Source: CAD feature listing. Evaluate the final solid. Frame: model axes, mm. Face numbers are marked on the shaded views. A direction names the side the tool comes from. Coordinates: 2 decimals unless noted, no trailing zeros. Order: outer loops, then holes, each group sorted by start corner. A loop starts at its lowest first (then second) coordinate and runs counter-clockwise, first axis right, second up.
```python
from build123d import *

# Parameters (mm, degrees)
SKETCH4_R           = 2
SKETCH4_R_2         = 3.96875
BOSS_EXTRUDE2_DEPTH = 6.35
FILLET1_R           = 5.08
FILLET7_R           = 3.81
FILLET9_R           = 5.08
FILLET10_R          = 1.27
FILLET11_R          = 3.81
FILLET12_R          = 2.54
FILLET13_R          = 3.81


with BuildPart() as part:
    # Sketch4 → Boss-Extrude2 (new body)
    with BuildSketch(Plane(origin=(0, 0, 0), x_dir=(1, 0, 0), z_dir=(0, 1, 0))):
        with BuildLine():
            Line((22.483900583, -18.4375), (28.735494078, -18.4375))
            Line((28.735494078, -18.4375), (48.985566477, 12.027918285))
            Line((48.985566477, 12.027918285), (54.680415238, 16.319294633))
            ThreePointArc((54.680415238, 16.319294633), (55.797199918, 17.662082259), (56.1975, 19.362095927))
            Line((56.1975, 19.362095927), (56.1975, 26.9875))
            ThreePointArc((56.1975, 26.9875), (55.081576836, 29.681576836), (52.3875, 30.7975))
            Line((52.3875, 30.7975), (-4.7625, 30.7975))
            ThreePointArc((-4.7625, 30.7975), (-7.456576836, 29.681576836), (-8.5725, 26.9875))
            Line((-8.5725, 26.9875), (-8.5725, 12.607500122))
            Line((-8.5725, 12.607500122), (-8.5725, 0.508))
            Line((-8.5725, 0.508), (-23.52171402, 0.508))
            Line((-23.52171402, 0.508), (-23.52171402, -9.652))
            Line((-23.52171402, -9.652), (-14.139296969, -9.652))
            Line((-14.139296969, -9.652), (-23.148009155, -20.371437257))
            Line((-23.148009155, -20.371437257), (-17.314513469, -25.273959881))
            Line((-17.314513469, -25.273959881), (-11.569090649, -18.4375))
            Line((-11.569090649, -18.4375), (22.483900583, -18.4375))
        make_face()
        with Locations(Location((-17.78, -19.905950726, 0), (0, 0, 270))):
            Circle(SKETCH4_R, mode=Mode.SUBTRACT)
        with BuildLine():
            ThreePointArc((-16.29541402, -4.572), (-20.572189245, -4.832151892), (-16.358479767, -4.055532442))
            ThreePointArc((-16.358479767, -4.055532442), (-16.311238795, -4.311848108), (-16.29541402, -4.572))
        make_face(mode=Mode.SUBTRACT)
        with BuildLine():
            ThreePointArc((-7.62, -15.8975), (-10.16, -13.3575), (-7.62, -10.8175))
            Line((-7.62, -10.8175), (12.7, -10.8175))
            Line((12.7, -10.8175), (12.7, -5.7375))
            ThreePointArc((12.7, -5.7375), (15.24, -3.1975), (17.78, -5.7375))
            Line((17.78, -5.7375), (17.78, -13.3575))
            Line((17.78, -13.3575), (17.78, -15.8975))
            Line((17.78, -15.8975), (15.24, -15.8975))
            Line((15.24, -15.8975), (-7.62, -15.8975))
        make_face(mode=Mode.SUBTRACT)
        with BuildLine():
            ThreePointArc((-6.163414949, -1.528010526), (-1.528010526, 6.163414949), (6.163414949, 1.528010526))
            ThreePointArc((6.163414949, 1.528010526), (6.303181138, 0.769680153), (6.35, 0))
            ThreePointArc((6.35, 0), (0.769680153, -6.303181138), (-6.163414949, -1.528010526))
        make_face(mode=Mode.SUBTRACT)
        with Locations(Location((24.012521227, -14.703599027, 0), (0, 0, 270))):
            Circle(SKETCH4_R, mode=Mode.SUBTRACT)
        with Locations(Location((-1.5875, 21.9075, 0), (0, 0, 270))):
            Circle(SKETCH4_R_2, mode=Mode.SUBTRACT)
        with BuildLine():
            ThreePointArc((20.58801402, 4.572), (18.701865912, 2.441524775), (16.358479767, 4.055532442))
            ThreePointArc((16.358479767, 4.055532442), (18.181562129, 6.702475225), (20.58801402, 4.572))
        make_face(mode=Mode.SUBTRACT)
        Polygon((6.749565973, 9.2075), (6.749565973, 26.9875), (40.692955064, 26.9875), (40.692955064, 7.472580753), (33.28904903, -3.666297657), (23.452955064, -3.666297657), (23.452955064, 9.2075), align=None, mode=Mode.SUBTRACT)
        with Locations(Location((49.2125, 21.9075, 0), (0, 0, 270))):
            Circle(SKETCH4_R_2, mode=Mode.SUBTRACT)
    extrude(amount=-BOSS_EXTRUDE2_DEPTH)

    # Fillet1
    fillet1_edges = [part.edges().sort_by_distance(p)[0] for p in [
        (48.985566477, -3.175, -12.027918285),
        (28.735494078, -3.175, 18.4375),
    ]]
    fillet(fillet1_edges, radius=FILLET1_R)

    # Fillet7
    fillet7_edges = [part.edges().sort_by_distance(p)[0] for p in [
        (40.692955064, -3.175, -7.472580753),
        (40.692955064, -3.175, -26.9875),
        (6.749565973, -3.175, -26.9875),
        (6.749565973, -3.175, -9.2075),
    ]]
    fillet(fillet7_edges, radius=FILLET7_R)

    # Fillet9
    fillet9_edges = [part.edges().sort_by_distance(p)[0] for p in [
        (-11.569090649, -3.175, 18.4375),
        (12.7, -3.175, 10.8175),
        (17.78, -3.175, 15.8975),
    ]]
    fillet(fillet9_edges, radius=FILLET9_R - 0.0001)  # a hair under: the kernel refuses the full size

    # Fillet10
    fillet10_edges = [part.edges().sort_by_distance(p)[0] for p in [
        (-14.139296969, -3.175, 9.652),
    ]]
    fillet(fillet10_edges, radius=FILLET10_R)

    # Fillet11
    fillet11_edges = [part.edges().sort_by_distance(p)[0] for p in [
        (-17.314513469, -3.175, 25.273959881),
        (-23.148009155, -3.175, 20.371437257),
    ]]
    fillet(fillet11_edges, radius=FILLET11_R - 0.0001)  # a hair under: the kernel refuses the full size

    # Fillet12
    fillet12_edges = [part.edges().sort_by_distance(p)[0] for p in [
        (23.452955064, -3.175, -9.2075),
        (23.452955064, -3.175, 3.666297657),
        (-23.52171402, -3.175, 9.652),
        (-23.52171402, -3.175, -0.508),
        (-8.5725, -3.175, -0.508),
    ]]
    fillet(fillet12_edges, radius=FILLET12_R)

    # Fillet13
    fillet13_edges = [part.edges().sort_by_distance(p)[0] for p in [
        (33.28904903, -3.175, 3.666297657),
    ]]
    fillet(fillet13_edges, radius=FILLET13_R)


solid = part.part
```
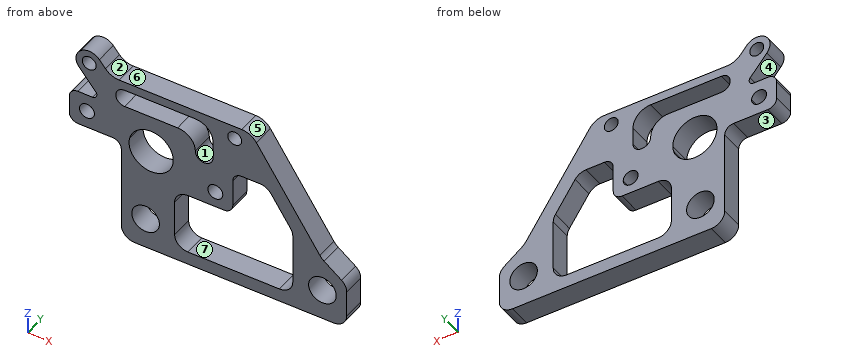
1. Pin query (flat end, axial travel): P1, Ø3, axis at y = -3.5, z = -14, coming from the -X side; P2, Ø1.9, axis at x = 28, y = -3, coming from the +Z side. Return the tip coordinate at first contact, or that it passes through.
Findings:
P1: stops at x = -8.57
P2: stops at z = 18.33
2. Section query A-A on x = -17.78. Return loops of the section in (y, z).
Findings:
outline: (-6.35, -0.51) - (0, -0.51) - (0, 2.53) - (-6.35, 2.53) - close; (-6.35, 6.61) - (0, 6.61) - (0, 9.65) - (-6.35, 9.65) - close; (-6.35, 13.98) - (0, 13.98) - (0, 17.91) - (-6.35, 17.91) - close; (-6.35, 21.91) - (0, 21.91) - (0, 23.72) - (-6.35, 23.72) - close
3. Access query for the marked faces 1, 2, 3 and 4. Directions: +Z, -Z, +X, -X, +Y, -Y. A direction counts if a zero-diameter tool reaches every point of the face in a straight line with its end or side. Return the directions, or none.
Findings:
face 1: +Y, -Y
face 2: +Z, +X, +Y, -Y
face 3: -Z, -X, +Y, -Y
face 4: -X, +Y, -Y
4. Ray query, line 1 (X direction, y = -5.5, z = -19); line 2 (X direction, y = -4.75, z = -3.5); line 3 (Z direction, x = 25.5, y = -2.75). Return the intervals inside material, ascending.
Findings:
line 1: x = -8.57 to -4.29, 1.11 to 6.75, 40.69 to 46.51, 51.91 to 56.18
line 2: x = -8.57 to -5.3, 5.3 to 16.58, 20.3 to 23.45, 38.05 to 43.32
line 3: z = -30.8 to -26.99, 3.62 to 13.37, 16.04 to 18.44
5. Section query D-D on z = -21.5. Return loops of the section in (x, y).
Findings:
outline: (-8.57, -6.35) - (-5.54, -6.35) - (-5.54, 0) - (-8.57, 0) - close; (2.36, -6.35) - (6.75, -6.35) - (6.75, 0) - (2.36, 0) - close; (40.69, -6.35) - (45.26, -6.35) - (45.26, 0) - (40.69, 0) - close; (53.16, -6.35) - (56.2, -6.35) - (56.2, 0) - (53.16, 0) - close
6. Section query B-B on z = 8.5. Return loops of the section in (x, y), plus the area to 3 significant figures.
Findings:
outline: (-23.11, -6.35) - (11.88, -6.35) - (11.88, 0) - (-23.11, 0) - close; (17.78, -6.35) - (35.34, -6.35) - (35.34, 0) - (17.78, 0) - close
area: 334 mm2
7. Section query C-C on x = 13.5. Return loops of the section in (y, z).
Findings:
outline: (-6.35, -30.8) - (0, -30.8) - (0, -26.99) - (-6.35, -26.99) - close; (-6.35, -9.21) - (0, -9.21) - (0, 3.89) - (-6.35, 3.89) - close; (-6.35, 15.83) - (0, 15.83) - (0, 18.44) - (-6.35, 18.44) - close
8. Draft query along X for the marked faces 5, 6 and 7. Return one class per face: released by +X, released by -X, zero draft, split by the parting line, or undercut.
Findings:
face 5: released by +X
face 6: zero draft
face 7: undercut
